from build123d import *

# Parameters (mm, degrees)
F0_R     = 1.5
F1_DEPTH = 10
F2_DEPTH = 5.25
F3_R     = 9
F3_R_2   = 7
F3_R_3   = 2.75
F4_DEPTH = 30
F5_DEPTH = 8.8
F6_DEPTH = 5.0771655029


# Not quite as in the source:
# - ends of sketch curves that miss each other by under 0.0002 mm in the source are joined


with BuildPart() as f1:
    # F0 (on Front) → F1 (new body, symmetric)
    with BuildSketch(Plane.XZ):
        with BuildLine():
            ThreePointArc((20.0087781194, -9.6635037267), (10.2175079385, -6.5385316067), (-0.005862, -5.4815880859))
            ThreePointArc((-0.005862, -5.4815880859), (-10.2228373041, -6.5359722724), (-20.0087868417, -9.6558283627))
            Line((-20.0087868417, -9.6558283627), (-20.008784, -29.496459))
            Line((-20.008784, -29.496459), (-20.008784, -29.500828))
            ThreePointArc((-20.008784, -29.500828), (-17.5087901054, -33.8309491846), (-12.5087967107, -33.8309485011))
            ThreePointArc((-12.5087967107, -33.8309485011), (-0.2003110708, -30.4823215942), (12.1580317725, -33.6419823498))
            ThreePointArc((12.1580317725, -33.6419823498), (12.4912575647, -33.830982099), (12.8215481384, -34.0250657685))
            ThreePointArc((12.8215481384, -34.0250657685), (17.6641901361, -33.7471454023), (20.008785, -29.500824))
            Line((20.008785, -29.500824), (20.0087781194, -9.6635037267))
        make_face()
        with Locations((-15.008794, -29.500828)):
            Circle(F0_R, mode=Mode.SUBTRACT)
        with Locations((-7.773364, -26.503811)):
            Circle(F0_R, mode=Mode.SUBTRACT)
        with BuildLine():
            ThreePointArc((-0.008573175, -23.9815880161), (1.0519448888, -24.4210055509), (1.491207, -25.481588))
            ThreePointArc((1.491207, -25.481588), (-1.0695308888, -26.5421704491), (-0.008573175, -23.9815880161))
        make_face(mode=Mode.SUBTRACT)
        with Locations((7.755782, -26.503815)):
            Circle(F0_R, mode=Mode.SUBTRACT)
        with Locations((14.991208, -29.500824)):
            Circle(F0_R, mode=Mode.SUBTRACT)
        with BuildLine():
            Line((-0.0051292502, -0.48159), (-0.0058619999, -5.4815880859))
            ThreePointArc((-0.0058619999, -5.4815880859), (10.2175079385, -6.5385316067), (20.0087781194, -9.6635037267))
            Line((20.0087781194, -9.6635037267), (20.008783, -4.481588))
            ThreePointArc((20.008783, -4.481588), (18.8372111247, -1.6531608753), (16.008784, -0.481588))
            Line((16.008784, -0.481588), (9.991212, -0.48159))
            Line((9.991212, -0.48159), (-0.0051292502, -0.48159))
        make_face()
        with BuildLine():
            ThreePointArc((-20.0087868417, -9.6558283627), (-10.2228373041, -6.5359722724), (-0.005862, -5.4815880859))
            Line((-0.005862, -5.4815880859), (-0.0051292502, -0.48159))
            Line((-0.0051292502, -0.48159), (-10.008792, -0.48159))
            Line((-10.008792, -0.48159), (-16.008784, -0.48159))
            ThreePointArc((-16.008784, -0.48159), (-18.8372111247, -1.6531608753), (-20.008784, -4.481588))
            Line((-20.008784, -4.481588), (-20.0087868417, -9.6558283627))
        make_face()
    extrude(amount=F1_DEPTH, both=True)

    # F0 (on Front) → F2 (cut, symmetric)
    with BuildSketch(Plane.XZ):
        with BuildLine():
            ThreePointArc((20.0087781194, -9.6635037267), (10.2175079385, -6.5385316067), (-0.005862, -5.4815880859))
            ThreePointArc((-0.005862, -5.4815880859), (-10.2228373041, -6.5359722724), (-20.0087868417, -9.6558283627))
            Line((-20.0087868417, -9.6558283627), (-20.008784, -29.496459))
            Line((-20.008784, -29.496459), (-20.008784, -29.500828))
            ThreePointArc((-20.008784, -29.500828), (-17.5087901054, -33.8309491846), (-12.5087967107, -33.8309485011))
            ThreePointArc((-12.5087967107, -33.8309485011), (-0.2003110708, -30.4823215942), (12.1580317725, -33.6419823498))
            ThreePointArc((12.1580317725, -33.6419823498), (12.4912575647, -33.830982099), (12.8215481384, -34.0250657685))
            ThreePointArc((12.8215481384, -34.0250657685), (17.6641901361, -33.7471454023), (20.008785, -29.500824))
            Line((20.008785, -29.500824), (20.0087781194, -9.6635037267))
        make_face()
        with Locations((-15.008794, -29.500828)):
            Circle(F0_R, mode=Mode.SUBTRACT)
        with Locations((-7.773364, -26.503811)):
            Circle(F0_R, mode=Mode.SUBTRACT)
        with BuildLine():
            ThreePointArc((-0.008573175, -23.9815880161), (1.0519448888, -24.4210055509), (1.491207, -25.481588))
            ThreePointArc((1.491207, -25.481588), (-1.0695308888, -26.5421704491), (-0.008573175, -23.9815880161))
        make_face(mode=Mode.SUBTRACT)
        with Locations((7.755782, -26.503815)):
            Circle(F0_R, mode=Mode.SUBTRACT)
        with Locations((14.991208, -29.500824)):
            Circle(F0_R, mode=Mode.SUBTRACT)
    extrude(amount=F2_DEPTH, both=True, mode=Mode.SUBTRACT)

    # F3 (on face) → F4 (join)
    with BuildSketch(Plane.XY.offset(-0.48159)):
        Circle(F3_R)
        Circle(F3_R_2, mode=Mode.SUBTRACT)
        Circle(F3_R_2)
        Polygon((3.8423572259, 2.4575647055), (4.0494920794, -2.0987966153), (0.2071348534, -4.5563613208), (-3.8423572259, -2.4575647055), (-4.0494920794, 2.0987966153), (-0.2071348534, 4.5563613208), align=None, mode=Mode.SUBTRACT)
        Polygon((0.2071348534, -4.5563613208), (4.0494920794, -2.0987966153), (3.8423572259, 2.4575647055), (-0.2071348534, 4.5563613208), (-4.0494920794, 2.0987966153), (-3.8423572259, -2.4575647055), align=None)
        Circle(F3_R_3, mode=Mode.SUBTRACT)
    extrude(amount=F4_DEPTH)

    # F3 (on face) → F5 (join)
    with BuildSketch(Plane.XY.offset(-0.48159)):
        Circle(F3_R_2)
        Polygon((3.8423572259, 2.4575647055), (4.0494920794, -2.0987966153), (0.2071348534, -4.5563613208), (-3.8423572259, -2.4575647055), (-4.0494920794, 2.0987966153), (-0.2071348534, 4.5563613208), align=None, mode=Mode.SUBTRACT)
    extrude(amount=-F5_DEPTH)

    # F3 (on face) → F6 (cut, through all)
    with BuildSketch(Plane.XY.offset(-0.48159)):
        Circle(F3_R_3)
    extrude(amount=-F6_DEPTH, mode=Mode.SUBTRACT)


solid = f1.part
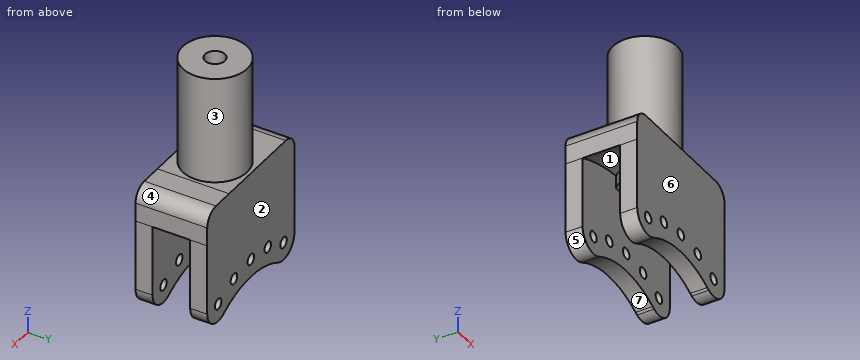
Can you work these out from the model? Positions are in its coordinate system, mm. Face numbers are marked on the shaded views. A direction names the side the tool comes from. Round coordinates to 2 decimals unless told otherwise and drop trailing zeros. Write each loop counter-clockwise with the first axis right and the second up, starting at its lowest first coordinate (ties: lowest second). Pieces come first, ordered by that corner, then holes. Notation, with made-up numbers: M 67.25,-36.5 L 81.25,-36.5 A17 ccw 81.25,-32.5 Z; hole C 35.25,32.25 d3. An arc over 180 degrees is marked long. Use a Markdown table: item, result.
Item 1: Which directions (+Z, -Z, +X, -X, +Y, -Y) give clear straight access to the entire face, cutting with the end or side of a thin tool? Please do the marked faces 1, 2 and 3.
Found:
| item | result |
|---|---|
| face 1 | -Z |
| face 2 | +Z, -Z, +X, -X, +Y |
| face 3 | +Z |
Item 2: We'd pull the mould along X, two halves only. Please class the marked faces 4, 5, 6 and 7: released by +X, released by -X, zero draft, split by the parting line, or undercut.
Found:
| item | result |
|---|---|
| face 4 | released by +X |
| face 5 | undercut |
| face 6 | zero draft |
| face 7 | undercut |
Item 3: I want a section at B-B (z = 14). List the corners of the cut face in (x, y) for me, and give its area (3 significant figures).
Found:
| item | result |
|---|---|
| outline | C 0,0 d18; hole C 0,0 d5.5 |
| area | 231 mm2 |
Item 4: I want a section at C-C (y = -3.75). List the corners of the cut face in (x, z) for me.
Found:
| item | result |
|---|---|
| outline | M -20.01,-9.66 A50 cw -5.91,-5.83 L -5.91,-9.28 L -1.35,-9.28 L -1.35,-5.5 A50 cw 1.47,-5.5 L 1.47,-9.28 L 5.91,-9.28 L 5.91,-5.83 A50 cw 20.01,-9.66 L 20.01,-4.48 A4 ccw 16.01,-0.48 L 9.99,-0.48 L 8.18,-0.48 L 8.18,29.52 L -8.18,29.52 L -8.18,-0.48 L -16.01,-0.48 A4 ccw -20.01,-4.48 Z |
Item 5: For pin 1 Ø2.5 at (x, z) = (-0.01, -25.48) entering from -Y; pin 2 Ø5.5 at (x, y) = (-3.5, 0) entering from -Z; pin 3 Ø10 at (x, z) = (2, 19) entering from -Y; pin 4 Ø1.5 at (x, y) = (-10.5, 2.5) entering from +Z, each with a flat end and sliding along its axis, tell me the tip position at first contact or that it passes through.
Found:
| item | result |
|---|---|
| pin 1 | passes through |
| pin 2 | stops at z = -9.28 |
| pin 3 | stops at y = -9 |
| pin 4 | stops at z = -0.48 |
Item 6: I want a section at A-A (y = 0). List the corners of the cut face in (x, z) for me.
Found:
| item | result |
|---|---|
| outline | M -20.01,-9.66 A50 cw -7,-5.97 L -7,-9.28 L -3.95,-9.28 L -3.95,-5.64 A50 cw -2.75,-5.56 L -2.75,29.52 L -9,29.52 L -9,-0.48 L -16.01,-0.48 A4 ccw -20.01,-4.48 Z; M 2.75,-5.56 A50 cw 3.95,-5.64 L 3.95,-9.28 L 7,-9.28 L 7,-5.98 A50 cw 20.01,-9.66 L 20.01,-4.48 A4 ccw 16.01,-0.48 L 9.99,-0.48 L 9,-0.48 L 9,29.52 L 2.75,29.52 Z |
Item 7: If I drill on line 1 along Y through (x, z) = (-12, -14); line 2 along Z through (x, y) = (5, -0.5), over which ranges is the centre line in solid material (lowest first)? Write a range as [from, to].
Found:
| item | result |
|---|---|
| line 1 | y = [-10, -5.25], [5.25, 10] |
| line 2 | z = [-9.28, 29.52] |
